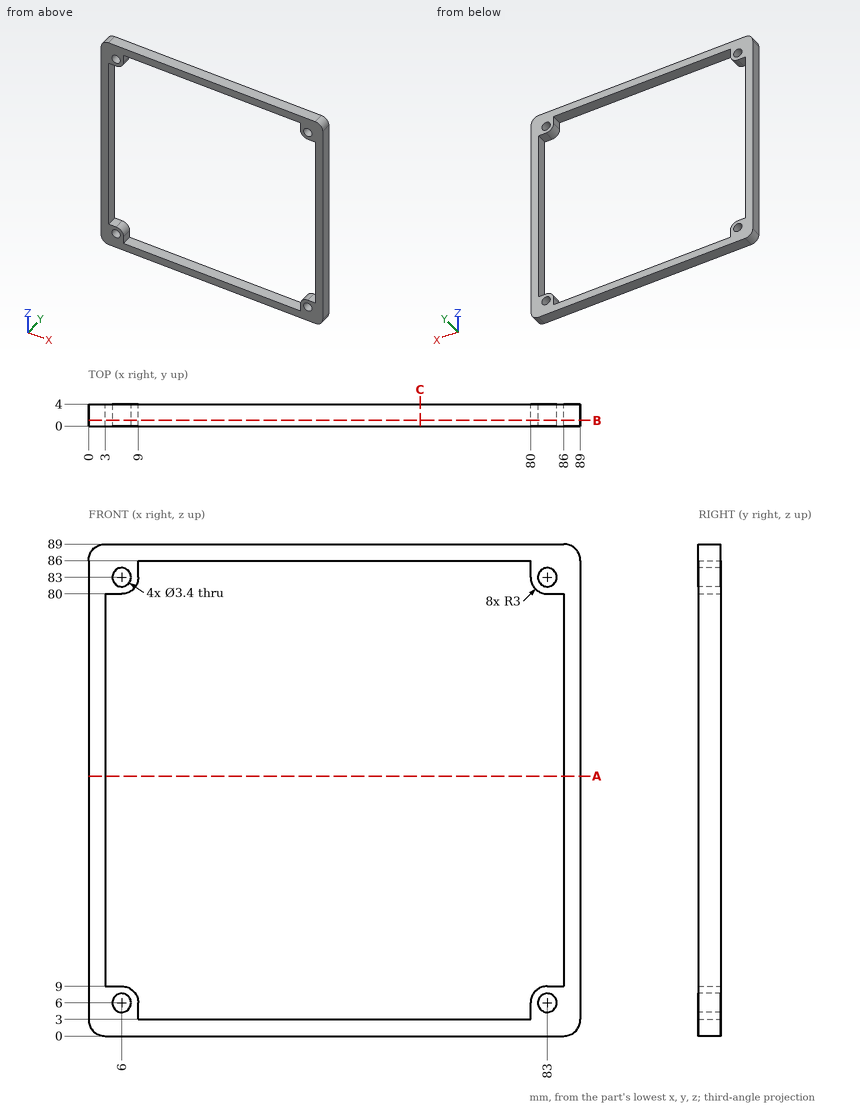
Study the drawing (mm; zero at the part's minimum x, y, z) and answer. Coordinates: 2 decimals unless noted, no trailing zeros. Loops run counter-clockwise (first coordinate to the right, second up) from the corner with the lowest first, then second, coordinate; pieces in that order, holes last. Notation, with made-up numbers: M 42,-15 L 101,-15 A10 ccw 101,-6 Z; hole C -29.5,6 d9. An arc over 180 degrees is marked long. Answer in a Markdown table with one row per item. Add a question column.
1. Find section C-C, the plane x = 60. Write down the section's boundary in (y, z), then the cut area to 3 significant figures.
2. Find section B-B, the plane y = 1.05. Write down the section's boundary in (x, z).
3. Consider L1, parallel to X at y = 2.15, z = 83; L2, parallel to Z at x = 61.5, y = 3.4. Determine where each line is inside the solid, lowest interval first.
4. Find section A-A, the plane z = 47. Write down the section's boundary in (x, y).
Reported:
| question | item | result |
|---|---|---|
| 1 | outline | M 0,0 L 4,0 L 4,3 L 0,3 Z; M 0,86 L 4,86 L 4,89 L 0,89 Z |
| 1 | area | 24.0 mm^2 |
| 2 | outline | M 0,3 A3 ccw 3,0 L 86,0 A3 ccw 89,3 L 89,86 A3 ccw 86,89 L 3,89 A3 ccw 0,86 Z; hole M 3,9 L 6,9 A3 cw 9,6 L 9,3 L 80,3 L 80,6 A3 cw 83,9 L 86,9 L 86,80 L 83,80 A3 cw 80,83 L 80,86 L 9,86 L 9,83 A3 cw 6,80 L 3,80 Z; hole C 6,6 d3.4; hole C 6,83 d3.4; hole C 83,6 d3.4; hole C 83,83 d3.4 |
| 3 | L1 | x = 0 to 4.3, 7.7 to 9, 80 to 81.3, 84.7 to 89 |
| 3 | L2 | z = 0 to 3, 86 to 89 |
| 4 | outline | M 0,0 L 3,0 L 3,4 L 0,4 Z; M 86,0 L 89,0 L 89,4 L 86,4 Z |
